Source: CAD feature listing. Evaluate the final solid. Frame: model axes, mm. A direction names the side the tool comes from. Give positions to 0.01 mm unless a question says otherwise; leave off trailing zeros. Loops run counter-clockwise (first coordinate to the right, second up) from the corner with the lowest first, then second, coordinate; pieces in that order, holes last. Notation, with made-up numbers: M 36.25,9 L 46.25,9 A24 ccw 46.25,30 Z; hole C -1.5,8.25 d8. An arc over 180 degrees is marked long. Answer in a Markdown table with one row per item.
```python
from build123d import *

# Parameters (mm, degrees)
ODGI_CIE_BAZOWE1_DEPTH             = 3
ODGI_CIE_KRAW_DZI1_STRIP_W         = 16
ODGI_CIE_KRAW_DZI1_STRIP_H         = 3
ODGI_CIE_KRAW_DZI1_STRIP_CUT_DEPTH = 124
ODGI_CIE_KRAW_DZI1_DEPTH           = 124
WYTNIJ_WYCI_GNI_CIE1_DEPTH         = 84
OTW_R_5_2_5_2_1_D                  = 5.2
OTW_R_4_2_4_2_1_D                  = 4.2
WYTNIJ_WYCI_GNI_CIE2_DEPTH         = 104.310212467
ZAOKR_GLENIE1_R                    = 2


# Sheet-metal steps are written as plain solids
with BuildPart() as part:
    # Szkic1 → Odgięcie bazowe1 (new body)
    with BuildSketch(Plane.XY):
        Polygon((30, -42), (30, -62), (0, -62), (0, 62), (30, 62), (30, 42), (18, 42), (18, -42), align=None)
    extrude(amount=-ODGI_CIE_BAZOWE1_DEPTH)

    # Odgięcie krawędzi1 strip (across the edge) → Odgięcie krawędzi1 strip cut (cut)
    with BuildSketch(Plane.XZ.offset(-62)):
        with Locations((-6, -1.5)):
            Rectangle(ODGI_CIE_KRAW_DZI1_STRIP_W, ODGI_CIE_KRAW_DZI1_STRIP_H)
    extrude(amount=ODGI_CIE_KRAW_DZI1_STRIP_CUT_DEPTH, mode=Mode.SUBTRACT)

    # Odgięcie krawędzi1 section (across the edge) → Odgięcie krawędzi1 (add)
    with BuildSketch(Plane.XZ.offset(-62)):
        with BuildLine():
            Line((-3, 2), (-3, 77))
            Line((-3, 77), (0, 77))
            Line((0, 77), (0, 2))
            ThreePointArc((0, 2), (0.585786438, 0.585786438), (2, 0))
            Line((2, 0), (2, -3))
            ThreePointArc((2, -3), (-1.535533906, -1.535533906), (-3, 2))
        make_face()
    extrude(amount=ODGI_CIE_KRAW_DZI1_DEPTH)

    # Szkic10 → Wytnij-wyciągnięcie1 (cut)
    with BuildSketch(Plane(origin=(0, 62, 0), x_dir=(1, 0, 0), z_dir=(0, 1, 0))):
        with BuildLine():
            Line((2, 0), (2, 3))
            ThreePointArc((2, 3), (-1.535533906, 1.535533906), (-3, -2))
            Line((-3, -2), (-3, -77))
            Line((-3, -77), (0, -77))
            Line((0, -77), (0, -2))
            ThreePointArc((0, -2), (0.585786438, -0.585786438), (2, 0))
        make_face()
    extrude(amount=-WYTNIJ_WYCI_GNI_CIE1_DEPTH, mode=Mode.SUBTRACT)

    # Otwór Ø5.2 (5.2)1 (through all)
    with Locations(Plane(origin=(16, -46, 0), x_dir=(1, 0, 0), z_dir=(0, 0, 1))):
        with Locations((0, 0), (0, 96)):
            Hole(OTW_R_5_2_5_2_1_D / 2)

    # Otwór Ø4.2 (4.2)1 (through all)
    with Locations(Plane(origin=(0, -49, 69), x_dir=(0, 0, 1), z_dir=(1, 0, 0))):
        with Locations((0, 0), (0, -10)):
            Hole(OTW_R_4_2_4_2_1_D / 2)

    # Szkic14 → Wytnij-wyciągnięcie2 (cut, through all)
    with BuildSketch(Plane(origin=(0, 0, 0), x_dir=(0, 0, -1), z_dir=(1, 0, 0))):
        with BuildLine():
            Line((-69, -46.9), (-44, -46.9))
            ThreePointArc((-44, -46.9), (-41.9, -49), (-44, -51.1))
            Line((-44, -51.1), (-69, -51.1))
            ThreePointArc((-69, -51.1), (-71.1, -49), (-69, -46.9))
        make_face()
        with BuildLine():
            Line((-69, -36.9), (-44, -36.9))
            ThreePointArc((-44, -36.9), (-41.9, -39), (-44, -41.1))
            Line((-44, -41.1), (-69, -41.1))
            ThreePointArc((-69, -41.1), (-71.1, -39), (-69, -36.9))
        make_face()
    extrude(amount=-WYTNIJ_WYCI_GNI_CIE2_DEPTH, mode=Mode.SUBTRACT)

    # Zaokrąglenie1
    zaokr_glenie1_edges = [part.edges().sort_by_distance(p)[0] for p in [
        (30, 62, -1.5),
        (30, 42, -1.5),
        (18, 42, -1.5),
        (18, -42, -1.5),
        (30, -42, -1.5),
        (30, -62, -1.5),
        (2, 62, -1.5),
        (-1.5, -62, 77),
        (-1.5, -22, 77),
    ]]
    fillet(zaokr_glenie1_edges, radius=ZAOKR_GLENIE1_R)


solid = part.part
```
Q1. Mould query, pull axis Y, two halves, no side actions, for faces 6 (the flat face through (24, 42, -1)), 7 (the flat face through (16, 62, -1)), 8 (the flat face through (30, -52, -1)), 9 (the flat face through (-1, -41.1, 56)). Classes: +Y half, -Y half, draft (parallel to the pull), parting line (faces both ways), or undercut.
Values follow:
| item | result |
|---|---|
| face 6 | undercut |
| face 7 | +Y half |
| face 8 | draft |
| face 9 | undercut |
Q2. Section query B-B (z = 66). Output: boundary loops of the cut face in (x, y), plus the area to 3 significant figures.
Values follow:
| item | result |
|---|---|
| outline | M -3,-62 L 0,-62 L 0,-51.1 L -3,-51.1 Z; M -3,-46.9 L 0,-46.9 L 0,-41.1 L -3,-41.1 Z; M -3,-36.9 L 0,-36.9 L 0,-22 L -3,-22 Z |
| area | 94.8 mm^2 |
Q3. Ray query, probe 1 along Y at (x, z) = (16, -2.35); probe 2 along Z at (x, y) = (12, -5). Return the intervals inside material, ascending. Write a range as from..to.
Values follow:
| item | result |
|---|---|
| probe 1 | -62..-48.6, -43.4..47.4, 52.6..62 |
| probe 2 | -3..0 |
Q4. Section query C-C (x = 23.5). Output: boundary loops of the cut face in (y, z).
Values follow:
| item | result |
|---|---|
| outline | M -62,-3 L -42,-3 L -42,0 L -62,0 Z; M 42,-3 L 62,-3 L 62,0 L 42,0 Z |
Q5. Reachability of faces 1 (the cylindrical face through (-1, -42, -2)), 2 (the flat face through (2, 20, -1)), 3 (the flat face through (18, 1, -1)), 4 (the flat face through (13, 1, 0)), 5 (the flat face through (-1, -46.9, 57)) from +Z, -Z, +X, -X, +Y, -Y: full face, straight path, thin tool, end or side. Return the list, or none.
Values follow:
| item | result |
|---|---|
| face 1 | -Z, -X, +Y, -Y |
| face 2 | +Z, -Z, -X, +Y |
| face 3 | +Z, -Z, +X |
| face 4 | +Z, +X, +Y, -Y |
| face 5 | +X, -X |
Q6. Contact query for flat-ended pins moving along their axis: pin 1 Ø7 at (x, y) = (16, -46) entering from +Z; pin 2 Ø1.5 at (y, z) = (8, -1) entering from -X; pin 3 Ø2.5 at (x, z) = (-1.5, 54) entering from +Y. Output: stop coordinate, or through.
Values follow:
| item | result |
|---|---|
| pin 1 | z = 0 |
| pin 2 | x = 2 |
| pin 3 | y = -22 |
Q7. Section query D-D (y = 33.5). Output: boundary loops of the cut face in (x, z).
Values follow:
| item | result |
|---|---|
| outline | M 2,-3 L 18,-3 L 18,0 L 2,0 Z |
Q8. Section query A-A (x = 16). Output: boundary loops of the cut face in (y, z), plus the area to 3 significant figures.
Values follow:
| item | result |
|---|---|
| outline | M -62,-3 L -48.6,-3 L -48.6,0 L -62,0 Z; M -43.4,-3 L 47.4,-3 L 47.4,0 L -43.4,0 Z; M 52.6,-3 L 62,-3 L 62,0 L 52.6,0 Z |
| area | 341 mm^2 |
